Source: CAD feature listing. Evaluate the final solid. Frame: model axes, mm. A direction names the side the tool comes from. Round coordinates to 2 decimals unless told otherwise and drop trailing zeros. Write each loop counter-clockwise with the first axis right and the second up, starting at its lowest first coordinate (ties: lowest second). Pieces come first, ordered by that corner, then holes. Notation, with made-up numbers: M 55.5,9 L 69.5,9 A35 ccw 69.5,44 Z; hole C -24,-14 d4. An arc over 180 degrees is marked long. Answer in a Markdown table with one row per item.
Autodesk Inventor part; units mm, degrees
ref_plane "Work Plane1" through (0, 0, 2) normal (0, 0, 1) x (1, 0, 0)
ref_plane "YZ Plane" through (0, 0, 0) normal (1, 0, 0) x (0, 1, 0)
ref_plane "XZ Plane" through (0, 0, 0) normal (0, 1, 0) x (-1, 0, 0)
sketch "Sketch1" plane through (0, 0, 0) normal (0, 0, 1) x (1, 0, 0)
  circle A0 centre (0, 0) radius 5.5
  dimension "d0" = 11
extrude "Extrusion1" add sketch "Sketch1" along normal blind 4
sketch "Sketch2" plane through (0, 0, 4) normal (0, 0, 1) x (1, 0, 0)
  circle A0 centre (0, 0) radius 2
  dimension "d3" = 4
extrude "Extrusion2" cut sketch "Sketch2" against normal blind 4
sketch "Sketch3" plane through (0, 0, 4) normal (0, 0, 1) x (1, 0, 0)
  circle A0 centre (0, 0) radius 2
  circle A1 centre (0, 0) radius 3
  circle A2 centre (0, 0) radius 4.75
  dimension "d6" = 1
  dimension "d7" = 9.5
extrude "Extrusion3" cut sketch "Sketch3" against normal blind 0.3 contours A2
ref_plane "Work Plane1" through (0, 0, 2) normal (0, 0, 1) x (1, 0, 0)
mirror "Mirror1" about plane through (0, 0, 2) normal (0, 0, 1) of "Extrusion3"
chamfer "Chamfer1" distance 0.15 angle 45 6 edges at (-4.75, 0, 4) (-3, 0, 4) (-3, 0, 0) (-4.75, 0, 0) (-5.5, 0, 4) (-5.5, 0, 0)
properties part number "roller bearing" material "Steel AISI 1118"
Q1. Material intervals for probe 1 along Y at (x, z) = (0, 0.25); probe 2 along Y at (x, z) = (0, 1.5); probe 3 along Z at (x, y) = (-3.75, -2), sorted ascending.
Solutions:
| item | result |
|---|---|
| probe 1 | y = -5.5 to -4.75, -3 to -2, 2 to 3, 4.75 to 5.5 |
| probe 2 | y = -5.5 to -2, 2 to 5.5 |
| probe 3 | z = 0.3 to 3.7 |
Q2. Access query for faces 1 (the flat face through (3, -1, 3.7)), 2 (the flat face through (-3, -1, 0.3)), 3 (the flat face through (1, 2, 0)). Directions: +Z, -Z, +X, -X, +Y, -Y. A direction counts if a zero-diameter tool reaches every point of the face in a straight line with its end or side. Return the directions, or none.
Solutions:
| item | result |
|---|---|
| face 1 | +Z |
| face 2 | -Z |
| face 3 | -Z, +X, -X, +Y, -Y |
Q3. Pull-direction query (Y, two-part tool) for faces 4 (the cylindrical face through (0, -2, 2)), 5 (the flat face through (1, 2, 4)), 6 (the cylindrical face through (-1.19, 5.37, 1.97)); classes: pulls with the +Y half, pulls with the -Y half, needs draft (parallel to the pull), parting line crosses it, or undercut.
Solutions:
| item | result |
|---|---|
| face 4 | undercut |
| face 5 | needs draft |
| face 6 | parting line crosses it |
Q4. Contact query for flat-ended pins moving along their axis: pin 1 Ø1 at (x, z) = (1.5, 3) entering from +Y; pin 2 Ø2 at (y, z) = (-3, 1.5) entering from +X. Output: stop coordinate, or through.
Solutions:
| item | result |
|---|---|
| pin 1 | stops at y = 5.41 |
| pin 2 | stops at x = 5.12 |
Q5. Section A-A (z = 0.6). Return loops of the section in (x, y).
Solutions:
| item | result |
|---|---|
| outline | C 0,0 d11; hole C 0,0 d4 |
